The listing builds one solid part. Answer for the finished solid, in the listing's coordinates (mm). Face numbers are marked on the shaded views. A direction names the side the tool comes from. Coordinates: 2 decimals unless noted, no trailing zeros. Loops run counter-clockwise (first coordinate to the right, second up) from the corner with the lowest first, then second, coordinate; pieces in that order, holes last. Notation, with made-up numbers: M 21,77.5 L 65,77.5 A14 ccw 65,96.5 Z; hole C 57.25,11.25 d5. An arc over 180 degrees is marked long. Answer as CSV lines item,"result". Start each with the question number.
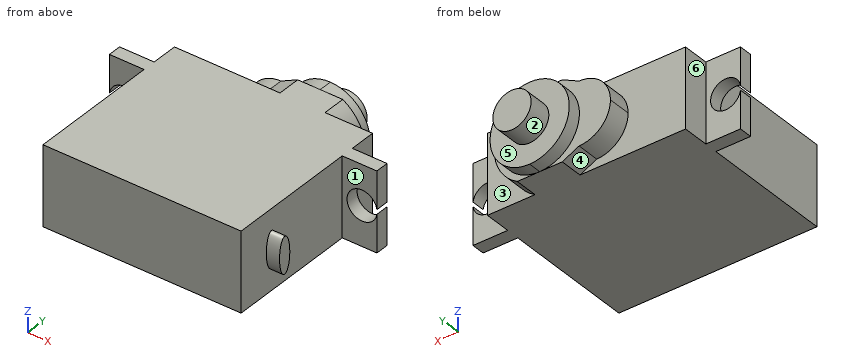
```python
from build123d import *

# Parameters (mm, degrees)
BOSS_EXTRUDE1_DEPTH = 12
SKETCH2_RX          = 2.776601092
SKETCH2_RY          = 1.017784095
BOSS_EXTRUDE2_DEPTH = 2
SKETCH3_R           = 2.275
CUT_EXTRUDE3_DEPTH  = 2
SKETCH5_R           = 2.9
BOSS_EXTRUDE3_DEPTH = 3.5
CUT_EXTRUDE4_DEPTH  = 5.5
CUT_EXTRUDE5_DEPTH  = 2
CUT_EXTRUDE6_DEPTH  = 3.5


with BuildPart() as part:
    # Sketch1 → Boss-Extrude1 (new body)
    with BuildSketch(Plane.XY):
        Polygon((0, 22), (0, 26), (8.7, 26), (8.7, 31.5), (26.3, 31.5), (26.3, 26), (30, 26), (30, 22), (35.25, 22), (35.25, 20), (30, 20), (30, 0), (0, 0), (0, 20), (-5.25, 20), (-5.25, 22), align=None)
    extrude(amount=BOSS_EXTRUDE1_DEPTH)

    # Sketch2 → Boss-Extrude2 (add)
    with BuildSketch(Plane(origin=(30, 0, 0), x_dir=(0, 0, -1), z_dir=(1, 0, 0))):
        with Locations((-6, 6)):
            Ellipse(SKETCH2_RX, SKETCH2_RY)
    extrude(amount=BOSS_EXTRUDE2_DEPTH)

    # Sketch3 → Cut-Extrude3 (cut)
    with BuildSketch(Plane(origin=(0, 22, 0), x_dir=(1, 0, 0), z_dir=(0, 1, 0))):
        with Locations((-3, -6)):
            Circle(SKETCH3_R)
        with Locations((33, -6)):
            Circle(SKETCH3_R)
    extrude(amount=-CUT_EXTRUDE3_DEPTH, mode=Mode.SUBTRACT)

    # Sketch5 → Boss-Extrude3 (add)
    with BuildSketch(Plane(origin=(0, 31.5, 0), x_dir=(1, 0, 0), z_dir=(0, 1, 0))):
        with Locations((19.4, -6)):
            Circle(SKETCH5_R)
    extrude(amount=BOSS_EXTRUDE3_DEPTH)

    # Sketch5<3> → Cut-Extrude4 (cut)
    with BuildSketch(Plane(origin=(0, 31.5, 0), x_dir=(1, 0, 0), z_dir=(0, 1, 0))):
        with BuildLine():
            Line((26.3, 0), (22.807345007, 0))
            ThreePointArc((22.807345007, 0), (25.363249137, -2.528738021), (26.3, -6))
            Line((26.3, -6), (26.3, 0))
        make_face()
        with BuildLine():
            Line((26.3, -12), (26.3, -6))
            ThreePointArc((26.3, -6), (25.363249137, -9.471261979), (22.807345007, -12))
            Line((22.807345007, -12), (26.3, -12))
        make_face()
    extrude(amount=-CUT_EXTRUDE4_DEPTH, mode=Mode.SUBTRACT)

    # Sketch7 → Cut-Extrude5 (cut)
    with BuildSketch(Plane(origin=(0, 31.5, 0), x_dir=(1, 0, 0), z_dir=(0, 1, 0))):
        with BuildLine():
            ThreePointArc((22.807345007, -12), (26.3, -6), (22.807345007, 0))
            Line((22.807345007, 0), (19.4, 0))
            ThreePointArc((19.4, 0), (23.642640687, -1.757359313), (25.4, -6))
            ThreePointArc((25.4, -6), (23.642640687, -10.242640687), (19.4, -12))
            Line((19.4, -12), (22.807345007, -12))
        make_face()
        with BuildLine():
            ThreePointArc((19.4, -12), (13.4, -6), (19.4, 0))
            Line((19.4, 0), (8.7, 0))
            Line((8.7, 0), (8.7, -12))
            Line((8.7, -12), (19.4, -12))
        make_face()
    extrude(amount=-CUT_EXTRUDE5_DEPTH, mode=Mode.SUBTRACT)

    # Sketch8 → Cut-Extrude6 (cut)
    with BuildSketch(Plane(origin=(0, 29.5, 0), x_dir=(1, 0, 0), z_dir=(0, 1, 0))):
        with BuildLine():
            Line((8.7, 0), (8.7, -6))
            ThreePointArc((8.7, -6), (10.091242789, -2.641242789), (13.45, -1.25))
            Line((13.45, -1.25), (15.992654993, 0))
            Line((15.992654993, 0), (8.7, 0))
        make_face()
        with BuildLine():
            Line((15.988961876, -12), (13.45, -10.75))
            ThreePointArc((13.45, -10.75), (10.091242789, -9.358757211), (8.7, -6))
            Line((8.7, -6), (8.7, -12))
            Line((8.7, -12), (15.988961876, -12))
        make_face()
    extrude(amount=-CUT_EXTRUDE6_DEPTH, mode=Mode.SUBTRACT)


solid = part.part
```
Item 1: Section C-C on x = 23.5 is taken. Determine the outline of the cut face in (y, z).
Item 2: Section B-B on y = 28.5 is taken. Determine the outline of the cut face in (x, z), then the cut area to 3 significant figures.
Item 3: For the marked faces 4, 5 and 6, determine the directions among +Z, -Z, +X, -X, +Y, -Y from which every point of the face is accessible in a straight line to the end or side of a thin tool.
Item 4: Section A-A on x = 33 is taken. Determine the outline of the cut face in (y, z) (3 decimals).
Item 5: For a pull along Y with two mould halves and no side action, classify the marked faces 1, 2 and 3 as pulls with the +Y half, pulls with the -Y half, needs draft (parallel to the pull), parting line crosses it, or undercut.
Item 6: Section D-D on z = 9.5 is taken. Determine the outline of the cut face in (x, y), then the cut area to 3 significant figures.
Item 7: Each of these flat-tipped pins is pushed along its axis until it touches: P1, Ø2, axis at x = 6.5, y = 8, coming from the -Z side; P2, Ø6, axis at y = 12.5, z = 2, coming from the +X side; P3, Ø2, axis at y = 24.5, z = 5.5, coming from the -X side; P4, Ø5.5, axis at x = 12.5, z = 7.5, coming from the +Y side. Where does it stop, or does it pass through?
Item 8: Consider line 1 (Z direction, x = -3, y = 20.6) (3 decimals); line 2 (X direction, y = 19.5, z = 2.5); line 3 (Y direction, x = 20.5, z = 11.25). Determine where each line is inside the solid, lowest interval first.
Results are:
1,outline,"M 0,0 L 26,0 L 26,0.45 L 29.5,0.45 L 29.5,1.62 L 31.5,1.62 L 31.5,10.38 L 29.5,10.38 L 29.5,11.55 L 26,11.55 L 26,12 L 0,12 Z"
2,outline,"M 13.45,1.25 L 15.99,0 L 22.81,0 A6.9 ccw 22.81,12 L 15.99,12 L 13.45,10.75 A4.75 ccw Z"
2,area,"174 mm²"
3,face 4,"-Z, -X, +Y"
3,face 5,"+Y"
3,face 6,"+Z, -Z, -X, +Y"
4,outline,"M 20,0 L 22,0 L 22,3.725 L 20,3.725 Z; M 20,8.275 L 22,8.275 L 22,12 L 20,12 Z"
5,face 1,"undercut"
5,face 2,"needs draft"
5,face 3,"pulls with the +Y half"
6,outline,"M -5.25,20 L 0,20 L 0,0 L 30,0 L 30,20 L 35.25,20 L 35.25,22 L 30,22 L 30,26 L 25.35,26 L 25.35,29.5 L 24.27,29.5 L 24.27,31.5 L 14.53,31.5 L 14.53,29.5 L 10.24,29.5 L 10.24,26 L 0,26 L 0,22 L -5.25,22 Z"
6,area,"873 mm²"
7,P1,"z = 0"
7,P2,"x = 30"
7,P3,"x = 0"
7,P4,"y = 31.5"
8,line 1,"0 to 3.725, 8.275 to 12"
8,line 2,"0 to 30"
8,line 3,"0 to 31.5"
